Verification items for the finished model (mm, model axes). A direction names the side the tool comes from. Give positions to 0.01 mm unless a question says otherwise; leave off trailing zeros. Order: outer loops, then holes, each group sorted by start corner. A loop starts at its lowest first (then second) coordinate and runs counter-clockwise, first axis right, second up. Notation, with made-up numbers: (-23.75, -39) -> (10.25, -39) arc R34 cw to (10.25, -7) -> close; hole circle Ø6 at (63, 78). An arc over 180 degrees is marked (long way). Write each question's results on one line, items separated by ' | '. Start each with the question number.
1. Material ranges on L1, parallel to Y at x = 0, z = 155.5; L2, parallel to Y at x = 60.5, z = 105; L3, parallel to X at y = 63, z = 200, recorded low to high. Write a range as from..to.
2. Set-up check for faces 1 (the face through (106, -106, 0)), 2 (the face through (-107.371, -483.522, 131.661)): record each of +Z, -Z, +X, -X, +Y, -Y from which the full face is reachable in a straight line by a thin tool's end or side.
3. Cross-section at A-A, the plane y = 0. Enter the section's corners in (x, z).
4. Mould release check, pull along Y, two halves, no side actions. Record for faces 3 (the face through (111, -487, 254)), 4 (the face through (-110.12, -495.92, 125.22)), 5 (the face through (-27.53, -123.98, 125.22)): +Y half, -Y half, draft (parallel to the pull), parting line (faces both ways), or undercut.
5. Cross-section at D-D, the plane y = -418. Enter the section's corners in (x, z).
6. Cross-section at C-C, the plane z = 208. Enter the section's corners in (x, y).
7. Depth check by flat-ended pin: pin 1 Ø5 at (y, z) = (-137.5, 32) entering from -X; pin 2 Ø2 at (y, z) = (220.5, 174) entering from -X; pin 3 Ø1 at (x, z) = (-270.5, 115) entering from -Y. Enter the tip coordinate at first touch or a pass-through.
from build123d import *

# Parameters (mm, degrees)
F0_R     = 508
F0_R_2   = 127
F1_DEPTH = 254
F2_T     = -12.7


with BuildPart() as f1:
    # F0 (on Top) → F1 (new body)
    with BuildSketch(Plane.XY):
        Circle(F0_R)
        Circle(F0_R_2, mode=Mode.SUBTRACT)
    extrude(amount=F1_DEPTH)

    # F2
    f2_openings = [f1.faces().sort_by_distance(p)[0] for p in [
        (-493.63159, 0, 254),
    ]]
    offset(amount=F2_T, openings=f2_openings)


solid = f1.part
Results below:
1) L1: y = -508..-495.3, -139.7..-127, 127..139.7, 495.3..508 | L2: y = -504.38..-491.59, -125.92..-111.66, 111.66..125.92, 491.59..504.38 | L3: x = -504.08..-491.28, -124.69..-110.27, 110.27..124.69, 491.28..504.08
2) face 1: -Z, +X, -X, +Y, -Y | face 2: +Z
3) outline: (-508, 0) -> (-127, 0) -> (-127, 254) -> (-139.7, 254) -> (-139.7, 12.7) -> (-495.3, 12.7) -> (-495.3, 254) -> (-508, 254) -> close; (127, 0) -> (508, 0) -> (508, 254) -> (495.3, 254) -> (495.3, 12.7) -> (139.7, 12.7) -> (139.7, 254) -> (127, 254) -> close
4) face 3: draft | face 4: parting line | face 5: undercut
5) outline: (-288.69, 0) -> (288.69, 0) -> (288.69, 254) -> (265.7, 254) -> (265.7, 12.7) -> (-265.7, 12.7) -> (-265.7, 254) -> (-288.69, 254) -> close
6) outline: circle Ø1016 at (0, 0); circle Ø279.4 at (0, 0); hole circle Ø990.6 at (0, 0); hole circle Ø254 at (0, 0)
7) pin 1: stops at x = -489.73 | pin 2: stops at x = -458.13 | pin 3: stops at y = -430.31
